from build123d import *

# Parameters (mm, degrees)
SKETCH1_R             = 6
SKETCH1_R_2           = 30
SKETCH1_R_3           = 12
BOSS_EXTRUDE1_DEPTH   = 20
BOSS_EXTRUDE2_DEPTH   = 7.5
BOSS_EXTRUDE2_2_DEPTH = 7.5
BOSS_EXTRUDE3_START   = -5
BOSS_EXTRUDE3_DEPTH   = 10


# Read off the part's stored shape, not the designer's step: Boss-Extrude3
with BuildPart() as part:
    # Sketch1 → Boss-Extrude1 (new body)
    # profile 1 of 2: a face of its own
    with BuildSketch(Plane.XY):
        with BuildLine():
            ThreePointArc((3.726717402, 29.767626331), (22.492237795, 19.851932877), (30, 0))
            ThreePointArc((30, 0), (22.492237795, -19.851932877), (3.726717402, -29.767626331))
            ThreePointArc((3.726717402, -29.767626331), (11.179632465, -31.260655735), (16.240407222, -36.931955285))
            ThreePointArc((16.240407222, -36.931955285), (34.277765833, -50.435016351), (55.021040607, -41.637544243))
            ThreePointArc((55.021040607, -41.637544243), (69, 0), (55.021040607, 41.637544243))
            ThreePointArc((55.021040607, 41.637544243), (34.277765833, 50.435016351), (16.240407222, 36.931955285))
            ThreePointArc((16.240407222, 36.931955285), (11.179632465, 31.260655735), (3.726717402, 29.767626331))
        make_face()
        with Locations((37, -28)):
            Circle(SKETCH1_R, mode=Mode.SUBTRACT)
        with Locations((37, 28)):
            Circle(SKETCH1_R, mode=Mode.SUBTRACT)
    # profile 2 of 2: a face of its own
    with BuildSketch(Plane.XY):
        Circle(SKETCH1_R_2)
        Circle(SKETCH1_R_3, mode=Mode.SUBTRACT)
    extrude(amount=-BOSS_EXTRUDE1_DEPTH)



with BuildPart() as body_2:
    # Sketch2 → Boss-Extrude2 (new, symmetric)
    with BuildSketch(Plane.XY.offset(-10)):
        with BuildLine():
            ThreePointArc((0, 75.029338215), (-20.696071905, 75.701090057), (-40.76800111, 70.612249245))
            ThreePointArc((-40.76800111, 70.612249245), (-47.155174797, 52.434957534), (-29.342215302, 45.092723837))
            ThreePointArc((-29.342215302, 45.092723837), (-28.949505146, 45.266435927), (-28.550831211, 45.42598608))
            ThreePointArc((-28.550831211, 45.42598608), (-27.650605488, 45.877879071), (-26.78520184, 46.393330477))
            ThreePointArc((-26.78520184, 46.393330477), (-13.82075983, 51.326021178), (0, 52.507034247))
            ThreePointArc((0, 52.507034247), (9.465684914, 63.768186231), (0, 75.029338215))
        make_face()
        with BuildLine():
            ThreePointArc((-28.954409532, 49.754065216), (-43.037682802, 53.155902064), (-38.942123297, 67.053292907))
            ThreePointArc((-38.942123297, 67.053292907), (-20.097629603, 71.750364494), (-0.687840355, 71.088922545))
            ThreePointArc((-0.687840355, 71.088922545), (5.465684914, 63.768186231), (-0.687840355, 56.447449916))
            ThreePointArc((-0.687840355, 56.447449916), (-15.317913255, 55.198724707), (-28.954409532, 49.754065216))
        make_face(mode=Mode.SUBTRACT)
    extrude(amount=BOSS_EXTRUDE2_DEPTH, both=True)


with BuildPart() as body_3:
    # Sketch2 → Boss-Extrude2 2 (new, symmetric)
    with BuildSketch(Plane.XY.offset(-10)):
        with BuildLine():
            ThreePointArc((-40.76800111, -70.612249245), (-20.696071905, -75.701090057), (0, -75.029338215))
            ThreePointArc((0, -75.029338215), (9.465684914, -63.768186231), (0, -52.507034247))
            ThreePointArc((0, -52.507034247), (-13.82075983, -51.326021178), (-26.78520184, -46.393330477))
            ThreePointArc((-26.78520184, -46.393330477), (-46.501784417, -51.155902064), (-40.76800111, -70.612249245))
        make_face()
        with BuildLine():
            ThreePointArc((-0.687840355, -56.447449916), (5.465684914, -63.768186231), (-0.687840355, -71.088922545))
            ThreePointArc((-0.687840355, -71.088922545), (-20.097629603, -71.750364494), (-38.942123297, -67.053292907))
            ThreePointArc((-38.942123297, -67.053292907), (-43.037682802, -53.155902064), (-28.954409532, -49.754065216))
            ThreePointArc((-28.954409532, -49.754065216), (-15.317913255, -55.198724707), (-0.687840355, -56.447449916))
        make_face(mode=Mode.SUBTRACT)
    extrude(amount=BOSS_EXTRUDE2_2_DEPTH, both=True)


with BuildPart() as part_1:
    add(part.part)

    add(body_2.part)  # Boss-Extrude3 merges body 2

    add(body_3.part)  # Boss-Extrude3 merges body 3
    # Boss-Extrude3 outline → Boss-Extrude3 (add)
    with BuildSketch(Plane.XY.offset(-10).offset(BOSS_EXTRUDE3_START)):
        with BuildLine():
            ThreePointArc((3.726717402, 29.767626331), (6.638008812, 29.759061772), (9.465684914, 30.451837991))
            Line((9.465684914, 30.451837991), (9.465684914, 63.768186231))
            ThreePointArc((9.465684914, 63.768186231), (6.784937065, 56.41269959), (0, 52.507034247))
            ThreePointArc((0, 52.507034247), (-13.820759831, 51.326021178), (-26.78520184, 46.393330477))
            ThreePointArc((-26.78520184, 46.393330477), (-12.59508777, 40.218032027), (-16.29220141, 25.190557223))
            ThreePointArc((-16.29220141, 25.190557223), (-6.68657143, 29.245337449), (3.726717402, 29.767626331))
        make_face()
        with BuildLine():
            ThreePointArc((3.726717402, -29.767626331), (-6.68657143, -29.245337449), (-16.29220141, -25.190557223))
            ThreePointArc((-16.29220141, -25.190557223), (-12.59508777, -40.218032027), (-26.78520184, -46.393330477))
            ThreePointArc((-26.78520184, -46.393330477), (-13.820759831, -51.326021178), (0, -52.507034247))
            ThreePointArc((0, -52.507034247), (6.784937065, -56.41269959), (9.465684914, -63.768186231))
            Line((9.465684914, -63.768186231), (9.465684914, -30.451837991))
            ThreePointArc((9.465684914, -30.451837991), (6.638008812, -29.759061772), (3.726717402, -29.767626331))
        make_face()
    extrude(amount=BOSS_EXTRUDE3_DEPTH)


solid = part_1.part
Work out the finished part from the listing and answer in its coordinate system (mm). A direction names the side the tool comes from. Round coordinates to 2 decimals unless told otherwise and drop trailing zeros. Write each loop counter-clockwise with the first axis right and the second up, starting at its lowest first coordinate (ties: lowest second). Pieces come first, ordered by that corner, then holes. Notation, with made-up numbers: (-16.75, 88.5) -> (31.25, 88.5) arc R31 cw to (31.25, 116.5) -> close; hole circle Ø8 at (-12.75, 36). An arc over 180 degrees is marked (long way). Write each question's results on one line, items separated by ' | '.
Item 1: Find the intervals of material crossed by line 1 along Y through (x, z) = (37, -11); line 2 along Y through (x, z) = (32.5, -1.75); line 3 along X through (y, z) = (-33, -9), in increasing order. Write a range as [from, to].
Result set:
line 1: [-50.6, -34], [-22, 22], [34, 50.6] | line 2: [-50.15, -31.97], [-24.03, 24.03], [31.97, 50.15] | line 3: [-11.5, 9.47], [13.51, 33.68], [40.32, 60.6]
Item 2: Flat-ended cylindrical pins translate along their axes: P1, Ø11, axis at x = -6.5, y = -35.5, coming from the +Z side; P2, Ø4, axis at y = -47, z = -3, coming from the +X side; P3, Ø6, axis at x = 54, z = -7, coming from the +Y side; P4, Ø5, axis at x = -15, y = -28, coming from the -Z side. Find the tip coordinate at first contact, or state that the pin passes through.
Result set:
P1: z = -5 | P2: x = 51.89 | P3: y = 45.74 | P4: z = -20
Item 3: The mould has two halves that part along Y. Classify faces 4 (the face through (9.466, -47, -10)), 5 (the face through (34, -50.4, -9.9)), 6 (the face through (-19.83, -71.78, -9.9)): +Y half, -Y half, draft (parallel to the pull), parting line (faces both ways), or undercut.
Result set:
face 4: draft | face 5: -Y half | face 6: undercut
Item 4: Which of the six approach directions +Z, -Z, +X, -X, +Y, -Y give full straight-line access (tool end or side, diameter ignored) to faces 1 (the face through (-1, 40, -15)), 2 (the face through (-20, 52, -2.5)), 3 (the face through (-15.52, -55.15, -9.9))?
Result set:
face 1: -Z | face 2: +Z, -X, +Y | face 3: +Z, -Z
Item 5: A cutting plane is placed at C-C, the plane x = -4. Count the separate pieces of the cut face and the enclosed holes in it, plus the area to 3 significant figures.
Result set:
separate pieces: 4 | enclosed holes: 0 | area: 1,430 mm^2
Item 6: A cutting plane is placed at B-B, the plane x = 37. Determine the outline of the cut face in (y, z), plus the area to 3 significant figures.
Result set:
outline: (-50.6, -20) -> (-34, -20) -> (-34, 0) -> (-50.6, 0) -> close; (-22, -20) -> (22, -20) -> (22, 0) -> (-22, 0) -> close; (34, -20) -> (50.6, -20) -> (50.6, 0) -> (34, 0) -> close | area: 1,540 mm^2
Item 7: A cutting plane is placed at A-A, the plane y = 0. Determine the outline of the cut face in (x, z), plus the area to 3 significant figures.
Result set:
outline: (-30, -20) -> (-12, -20) -> (-12, 0) -> (-30, 0) -> close; (12, -20) -> (69, -20) -> (69, 0) -> (12, 0) -> close | area: 1,500 mm^2
